Could you check a few things on this model? Use its own coordinates, in mm. A direction names the side the tool comes from. Coordinates: 2 decimals unless noted, no trailing zeros. Loops run counter-clockwise (first coordinate to the right, second up) from the corner with the lowest first, then second, coordinate; pieces in that order, holes last. Notation, with made-up numbers: (48, -5.5) - (100, -5.5) arc R16 ccw to (100, 25.5) - close; hole circle Ø6 at (75.5, -3.75). An arc over 180 degrees is marked (long way). Use CSV: the item, a comma, the result in double quotes.
from build123d import *

# Parameters (mm, degrees)
F0_R     = 3.175
F0_R_2   = 3.6159437641
F1_DEPTH = 3.048


with BuildPart() as f1:
    # F0 (on Front) → F1 (new body)
    with BuildSketch(Plane.XZ):
        with BuildLine():
            ThreePointArc((-9.525, 114.3), (0, 104.775), (9.525, 114.3))
            ThreePointArc((9.525, 114.3), (0, 123.825), (-9.525, 114.3))
        make_face()
        with Locations((0, 114.3)):
            Circle(F0_R, mode=Mode.SUBTRACT)
        with BuildLine():
            Line((15.3865384615, 67.4076923077), (9.525, 114.3))
            ThreePointArc((9.525, 114.3), (0, 104.775), (-9.525, 114.3))
            Line((-9.525, 114.3), (-15.3865384615, 67.4076923077))
            ThreePointArc((-15.3865384615, 67.4076923077), (0, 79.375), (15.3865384615, 67.4076923077))
        make_face()
        with Locations((-3.1260617511, 99.8911798788)):
            Circle(F0_R, mode=Mode.SUBTRACT)
        with BuildLine():
            Line((15.875, 63.5), (15.3865384615, 67.4076923077))
            ThreePointArc((15.3865384615, 67.4076923077), (0, 79.375), (-15.3865384615, 67.4076923077))
            Line((-15.3865384615, 67.4076923077), (-15.875, 63.5))
            Line((-15.875, 63.5), (-15.6509715667, 60.8424232807))
            ThreePointArc((-15.6509715667, 60.8424232807), (0, 47.625), (15.6509715667, 60.8424232807))
            Line((15.6509715667, 60.8424232807), (15.875, 63.5))
        make_face()
        with Locations((0, 63.5)):
            Circle(F0_R_2, mode=Mode.SUBTRACT)
        with BuildLine():
            ThreePointArc((15.875, 63.5), (15.7524112928, 65.4690514116), (15.3865384615, 67.4076923077))
            Line((15.3865384615, 67.4076923077), (15.875, 63.5))
        make_face()
        with BuildLine():
            Line((-15.875, 63.5), (-15.3865384615, 67.4076923077))
            ThreePointArc((-15.3865384615, 67.4076923077), (-15.7524112928, 65.4690514116), (-15.875, 63.5))
        make_face()
        with BuildLine():
            ThreePointArc((15.6509715667, 60.8424232807), (15.8188937448, 62.1664987103), (15.875, 63.5))
            Line((15.875, 63.5), (15.6509715667, 60.8424232807))
        make_face()
        with BuildLine():
            Line((-15.6509715667, 60.8424232807), (-15.875, 63.5))
            ThreePointArc((-15.875, 63.5), (-15.8188937448, 62.1664987103), (-15.6509715667, 60.8424232807))
        make_face()
        with BuildLine():
            Line((12.0396887444, 18.0029452157), (15.6509715667, 60.8424232807))
            ThreePointArc((15.6509715667, 60.8424232807), (0, 47.625), (-15.6509715667, 60.8424232807))
            Line((-15.6509715667, 60.8424232807), (-10.5220762583, 0))
            ThreePointArc((-10.5220762583, 0), (0, 10.5220762583), (10.5220762583, 0))
            ThreePointArc((10.5220762583, 0), (7.8595738312, -6.99579788), (1.2195038808, -10.4511673545))
            Line((1.2195038808, -10.4511673545), (44.45, -7.9375))
            ThreePointArc((44.45, -7.9375), (36.5125, 0), (44.45, 7.9375))
            Line((44.45, 7.9375), (19.4970935517, 9.3985203982))
            ThreePointArc((19.4970935517, 9.3985203982), (13.9539931587, 12.1282046514), (12.0396887444, 18.0029452157))
        make_face()
        with BuildLine():
            ThreePointArc((10.5220762583, 0), (0, 10.5220762583), (-10.5220762583, 0))
            ThreePointArc((-10.5220762583, 0), (-7.4402314744, -7.4402314744), (0, -10.5220762583))
            Line((0, -10.5220762583), (1.2195038808, -10.4511673545))
            ThreePointArc((1.2195038808, -10.4511673545), (7.8595738312, -6.99579788), (10.5220762583, 0))
        make_face()
        Circle(F0_R, mode=Mode.SUBTRACT)
        with BuildLine():
            Line((1.2195038808, -10.4511673545), (0, -10.5220762583))
            ThreePointArc((0, -10.5220762583), (0.6107818326, -10.504334074), (1.2195038808, -10.4511673545))
        make_face()
        with BuildLine():
            ThreePointArc((52.3875, 0), (50.0626600757, 5.6126600757), (44.45, 7.9375))
            ThreePointArc((44.45, 7.9375), (36.5125, 0), (44.45, -7.9375))
            ThreePointArc((44.45, -7.9375), (50.0626600757, -5.6126600757), (52.3875, 0))
        make_face()
        with Locations((44.45, 0)):
            Circle(F0_R, mode=Mode.SUBTRACT)
    extrude(amount=F1_DEPTH)


solid = f1.part
(1) Suppose I cut it at C-C (x = 37). Write out the boundary of the cut face in (y, z).
Computed:
outline,"(-3.05, -8.37) - (0, -8.37) - (0, 8.37) - (-3.05, 8.37) - close"
(2) Please list where these lines run through material, in increasing order: line 1 (X direction, y = -1.2, z = 114.5); line 2 (Z direction, x = 45, y = -2); line 3 (X direction, y = -1.55, z = 114).
Computed:
line 1,"x = -9.52 to -3.17, 3.17 to 9.52"
line 2,"z = -7.92 to -3.13, 3.13 to 7.92"
line 3,"x = -9.56 to -3.16, 3.16 to 9.56"
(3) Thinking about a two-plate mould opening in X: for faces 3 (the face through (3, 0, 43)), 4 (the face through (41.28, -1.5, 0.14)), 5 (the face through (-12.415, -1.503, 91.182)), which applies, +X half, -X half, draft (parallel to the pull), parting line (faces both ways), or undercut?
Computed:
face 3,"draft"
face 4,"undercut"
face 5,"-X half"
(4) Which directions (+Z, -Z, +X, -X, +Y, -Y) give clear straight access to the entire face, cutting with the end or side of a thin tool? Please do faces 1 (the face through (14.013, -1.503, 12.061)), 2 (the face through (-0.78, -1.5, 59.97)).
Computed:
face 1,"+X, +Y, -Y"
face 2,"+Y, -Y"
(5) Suppose I cut it at B-B (z = 90.5). Write out the boundary of the cut face in (x, y).
Computed:
outline,"(-12.5, -3.05) - (12.5, -3.05) - (12.5, 0) - (-12.5, 0) - close"
(6) Suppose I cut it at A-A (y = -2.5). State how many separate pieces and enclosed holes the cut face has, plus the area to 3 significant figures.
Computed:
separate pieces,"1"
enclosed holes,"5"
area,"3,850 mm²"
